For this review, use the dimensioned drawing (mm, ordinates from the lowest corner) and the shaded views. A direction names the side the tool comes from. Round coordinates to 2 decimals unless told otherwise and drop trailing zeros. Write each loop counter-clockwise with the first axis right and the second up, starting at its lowest first coordinate (ties: lowest second). Pieces come first, ordered by that corner, then holes. Notation, with made-up numbers: M 22.5,-21 L 29.5,-21 A30 cw 29.5,6 Z; hole C -9,41.5 d1. An arc over 180 degrees is marked long. One line per question, with ' | ' between items. Start each with the question number.
Item 1: Add section B-B, the plane z = 13.25. State the section outline as (x, y) points.
Item 2: Add section D-D, the plane x = 3.81. State the section outline as (y, z) points (1 decimal).
Item 3: Insertion check: pin 1 Ø8 at (x, z) = (3.81, 18.775) entering from +Y. The pin has a flat end and moves straight along its axis. Give the tip position at first contact, or say it passes through.
Item 4: For L1, parallel to Z at x = 22.5, y = 1.55 (3 decimals); L2, parallel to X at y = 3.8, z = 15.25; L3, parallel to X at y = 4.55, z = 8, list the stretches that pass through material, from the lowest coordinate up.
Item 5: Add section C-C, the plane z = 7.5. State the section outline as (x, y) points.
Item 6: Machinability: for the marked faces 1 and 2, which of the approach directions +Z, -Z, +X, -X, +Y, -Y give a long, thin tool a straight path to every point of the face, cutting with its end or side? Answer none if there is none.
Item 7: Draft analysis for pull direction X (two halves, no side actions). For the marked faces 3, 4, 5 and 6, state which applies: released by +X, released by -X, zero draft, split by the parting line, or undercut.
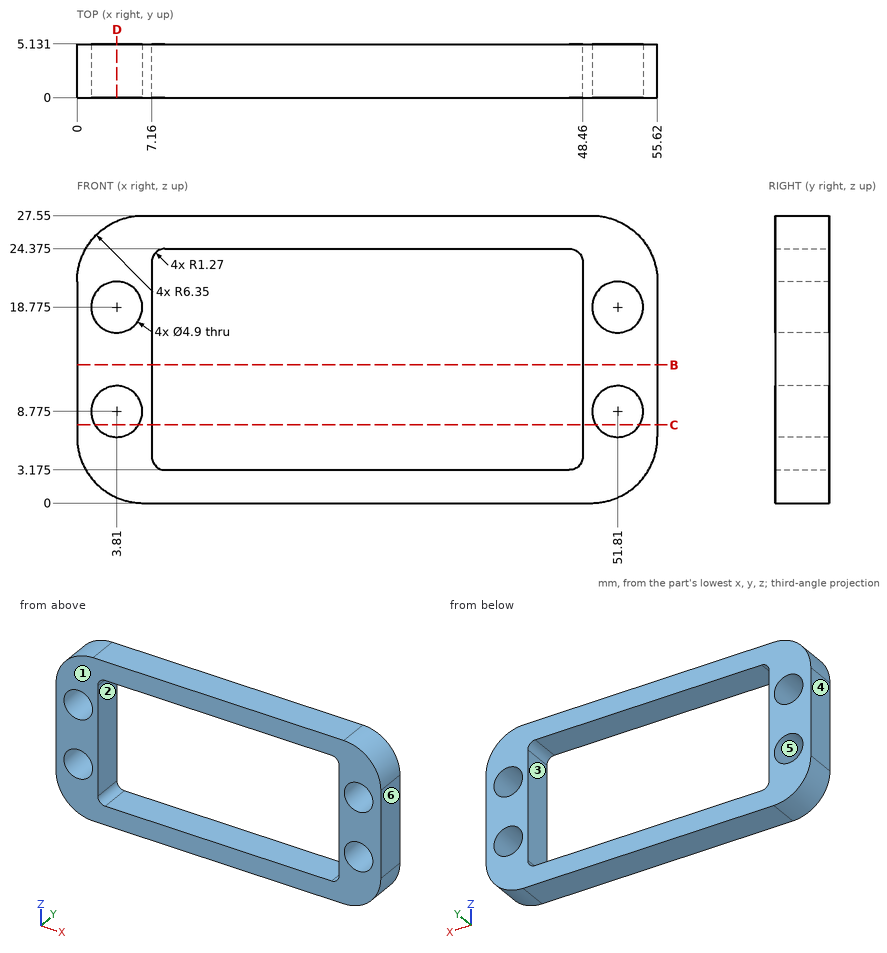
Computed values:
1) outline: M 0,0 L 7.16,0 L 7.16,5.13 L 0,5.13 Z; M 48.46,0 L 55.62,0 L 55.62,5.13 L 48.46,5.13 Z
2) outline: M 0,0.5 L 5.1,0.5 L 5.1,6.3 L 0,6.3 Z; M 0,11.2 L 5.1,11.2 L 5.1,16.3 L 0,16.3 Z; M 0,21.2 L 5.1,21.2 L 5.1,27 L 0,27 Z
3) pin 1: stops at y = 5.13
4) L1: z = 0 to 3.175, 24.375 to 27.55 | L2: x = 0 to 7.16, 48.46 to 55.62 | L3: x = 0 to 1.49, 6.13 to 7.16, 48.46 to 49.49, 54.13 to 55.62
5) outline: M 0,0 L 1.72,0 L 1.72,5.13 L 0,5.13 Z; M 5.9,0 L 7.16,0 L 7.16,5.13 L 5.9,5.13 Z; M 48.46,0 L 49.72,0 L 49.72,5.13 L 48.46,5.13 Z; M 53.9,0 L 55.62,0 L 55.62,5.13 L 53.9,5.13 Z
6) face 1: +Z, -Z, +X, -X, -Y | face 2: +Y, -Y
7) face 3: undercut | face 4: released by -X | face 5: undercut | face 6: released by +X
